Could you check a few things on this model? Use its own coordinates, in mm. Coordinates: 2 decimals unless noted, no trailing zeros. Loops run counter-clockwise (first coordinate to the right, second up) from the corner with the lowest first, then second, coordinate; pieces in that order, holes last.
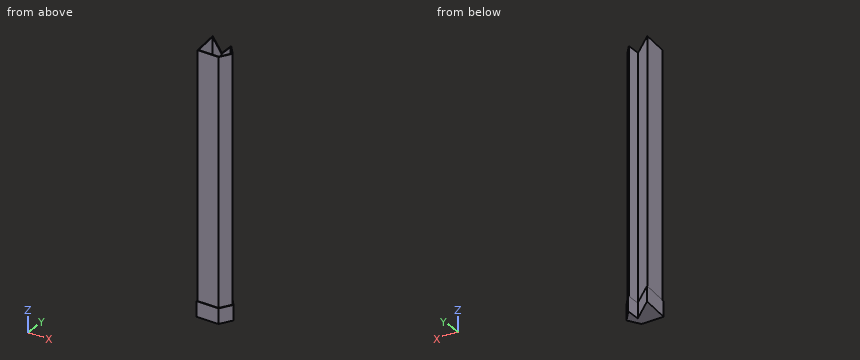
from build123d import *

# Parameters (mm, degrees)
F1_DEPTH = 56.642
F2_T     = -2.54
F3_DEPTH = 964.946
F4_T     = -2.54
F5_DEPTH = 25.4


with BuildPart() as f1:
    # F0 (on Top) → F1 (new body)
    with BuildSketch(Plane.XY):
        Polygon((-67.4327090383, 58.0582357943), (-57.1041107178, -52.6384785771), (26.6108643264, -53.1400032341), (53.9143458009, -8.2113463432), (17.0889906585, 37.5968702137), (17.0889906585, -17.2638874501), align=None)
    extrude(amount=F1_DEPTH)

    # F2
    f2_openings = [f1.faces().sort_by_distance(p)[0] for p in [
        (-14.363831, -12.367538, 56.642),
    ]]
    offset(amount=F2_T, openings=f2_openings, kind=Kind.INTERSECTION)

    # F3 (add): a face of the model
    f3_faces = [f1.faces().sort_by_distance(p)[0] for p in [
        (-14.8087693104, -13.6414291388, 2.54),
    ]]
    extrude(f3_faces, amount=F3_DEPTH)

    # F4
    f4_openings = [f1.faces().sort_by_distance(p)[0] for p in [
        (-14.808769, -13.641429, 967.486),
    ]]
    offset(amount=F4_T, openings=f4_openings, kind=Kind.INTERSECTION)

    # F0 (on Top) + F4_face (on face) → F5 (join)
    with BuildSketch(Plane.XY):
        Polygon((-67.4327090383, 58.0582357943), (-57.1041107178, -52.6384785771), (26.6108643264, -53.1400032341), (53.9143458009, -8.2113463432), (17.0889906585, 37.5968702137), (17.0889906585, -17.2638874501), align=None)
    with BuildSketch(Plane(origin=(-14.8087693104, -13.6414291388, 2.54), x_dir=(1, 0, 0), z_dir=(0, 0, 1))):
        Polygon((34.4377599689, -9.2882337449), (-49.4953159873, 65.509333201), (-39.980014566, -36.4708746559), (39.9961774627, -36.950000789), (65.6274259115, 5.2269490011), (34.4377599689, 44.024754652), align=None)
    extrude(amount=F5_DEPTH)


solid = f1.part
(1) For pin 1 (5 mm diameter, centred on y = -41.5, z = 261, fed in from +X); pin 2 (2 mm diameter, centred on x = 12, z = 480.5, fed in from +Y); pin 3 (8 mm diameter, centred on y = -32.5, z = 716.5, fed in from -X), each with a flat end and sliding along its axis, tell me the tip position at first contact or that it passes through.
Answers:
pin 1: stops at x = 32.23
pin 2: stops at y = -15.24
pin 3: stops at x = -56.81
(2) Imagine slicing it at D-D, the plane y = -37. Write out the boundary of the cut face in (x, z), and give its area (3 significant figures).
Answers:
outline: (-58.56, 0) - (36.42, 0) - (36.42, 56.64) - (33.45, 56.64) - (33.45, 967.49) - (30.47, 967.49) - (30.47, 54.1) - (33.45, 54.1) - (33.45, 27.94) - (-56.01, 27.94) - (-56.01, 54.1) - (-53.46, 54.1) - (-53.46, 967.49) - (-56.01, 967.49) - (-56.01, 56.64) - (-58.56, 56.64) - close
area: 7,860 mm2
(3) I need wall thicknesses on probe 1 along X at (y, z) = (-28, 652.5); probe 2 along X at (y, z) = (-20, 141.5); probe 3 along X at (y, z) = (13, 443.5). Which ranges of each line are inside material? Lowest first, please.
Answers:
probe 1: x = -56.85 to -54.3, 21.5 to 22.17, 35.94 to 38.92
probe 2: x = -57.6 to -55.05, 12.52 to 16.34, 19.63 to 22.17, 40.81 to 43.78
probe 3: x = -60.68 to -58.13, -24.51 to -20.69, 19.63 to 22.17, 30.34 to 33.6
(4) Imagine slicing it at C-C, the plane x = -22.5. Write out the boundary of the cut face in (y, z).
Answers:
outline: (-52.85, 0) - (18.02, 0) - (18.02, 56.64) - (14.61, 56.64) - (14.61, 967.49) - (11.21, 967.49) - (11.21, 54.1) - (14.61, 54.1) - (14.61, 27.94) - (-50.31, 27.94) - (-50.31, 54.1) - (-47.77, 54.1) - (-47.77, 967.49) - (-50.31, 967.49) - (-50.31, 56.64) - (-52.85, 56.64) - close
(5) Imagine slicing it at A-A, the plane z = 500. Write out the boundary of the cut face in (x, y), and give its area (3 significant figures).
Answers:
outline: (-64.3, 51.87) - (-54.79, -50.11) - (25.19, -50.59) - (50.82, -8.41) - (19.63, 30.38) - (19.63, -22.93) - close; hole (-61.18, 45.68) - (-52.47, -47.59) - (23.76, -48.04) - (47.72, -8.62) - (22.17, 23.17) - (22.17, -28.6) - close
area: 1,100 mm2
